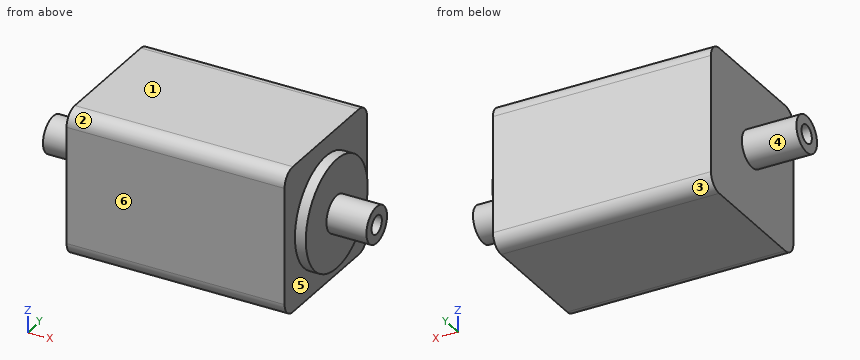
Autodesk Inventor part; units mm, degrees
ref_plane "Work Plane1" through (7, 10, -10) normal (1, 0, 0) x (0, 0, -1)
ref_plane "YZ Plane" through (0, 0, 0) normal (1, 0, 0) x (0, 1, 0)
ref_plane "XZ Plane" through (0, 0, 0) normal (0, 1, 0) x (-1, 0, 0)
sketch "Sketch1" plane through (0, 0, 0) normal (0, 1, 0) x (-1, 0, 0)
  line L0 (0, 0) -> (0, -20)
  line L1 (0, -20) -> (30, -20)
  line L2 (30, -20) -> (30, 0)
  line L3 (30, 0) -> (0, 0)
  dimension "d0" = 20
  dimension "d1" = 30
  dimension "d2" = 20
extrude "Extrusion1" add sketch "Sketch1" along normal blind 20
sketch "Sketch2" plane through (0, 0, 0) normal (1, 0, 0) x (0, 0, -1)
  line L0 (0, 0) -> (20, 0)
  line L1 (10, 0) -> (10, 10)
  circle A0 centre (10, 10) radius 7.5
  dimension "d5" = 10
  dimension "d6" = 15
extrude "Extrusion2" add sketch "Sketch2" along normal blind 1.5
sketch "Sketch3" plane through (1.5, 10, -10) normal (1, 0, 0) x (0, 0, -1)
  circle A0 centre (0, 0) radius 2.5
  point P0 (-10, -10)
  dimension "d9" = 5
extrude "Extrusion4" add sketch "Sketch3" along normal blind 5.5
sketch "Sketch4" plane through (-30, 0, -20) normal (-1, 0, 0) x (0, 0, 1)
  line L0 (20, 0) -> (0, 0)
  circle A0 centre (10, 10) radius 2.5
  circle A1 centre (10, 10) radius 2.5
  dimension "d16" = 5
extrude "Extrusion5" add sketch "Sketch4" along normal blind 7.5
sketch "Sketch5" plane through (-37.5, 10, -10) normal (-1, 0, 0) x (0, 0, 1)
  circle A0 centre (0, 0) radius 2.5
  point P0 (10, -10)
  dimension "d19" = 5
hole "Hole1" at (-37.5, 10, -10) direction (1, 0, 0) diameter 2.5 end through all
fillet "Fillet1" radius 2 4 edges at (-15, 20, -20) (-15, 20, 0) (-15, 0, -20) (-15, 0, 0)
ref_plane "Work Plane1" through (7, 10, -10) normal (1, 0, 0) x (0, 0, -1)
properties part number "NEMA8"
Read the model definition and answer for the solid it produces. Units are mm, in the model's axes. Face numbers are marked on the shaded views. A direction names the side the tool comes from. Give positions to 0.01 mm unless a question says otherwise; leave off trailing zeros. Loops run counter-clockwise (first coordinate to the right, second up) from the corner with the lowest first, then second, coordinate; pieces in that order, holes last.
Item 1: The part is cut by section D-D (y = 4). Write down the section's boundary in (x, z).
Item 2: The part is cut by section B-B (x = -26). Write down the section's boundary in (y, z), and give its area (3 significant figures).
Item 3: For the marked faces 4, 5 and 6, determine the directions among +Z, -Z, +X, -X, +Y, -Y from which every point of the face is accessible in a straight line to the end or side of a thin tool.
Item 4: The part is cut by section C-C (y = 10). Write down the section's boundary in (x, z), and give its area (3 significant figures).
Item 5: The mould has two halves that part along Y. Classify the marked faces 1, 2 and 3: released by +Y, released by -Y, zero draft, split by the parting line, or undercut.
Item 6: The part is cut by section A-A (z = -10). Write down the section's boundary in (x, y).
Item 7: Find the intervals of material crossed by line 1 along Y through (x, z) = (-9.5, -10); line 2 along Z through (x, y) = (-26, 10); line 3 along X through (y, z) = (4.5, -2), in increasing order.
Item 8: This flat-tipped pin is pushed along its axis until it touches: pin 1 Ø6 at (y, z) = (2.5, -8) entering from +X. Where does it stop, or does it pass through?
Taken from the geometry:
1. outline: (-30, -20) - (0, -20) - (0, -14.5) - (1.5, -14.5) - (1.5, -5.5) - (0, -5.5) - (0, 0) - (-30, 0) - close
2. outline: (0, -18) arc R2 ccw to (2, -20) - (18, -20) arc R2 ccw to (20, -18) - (20, -2) arc R2 ccw to (18, 0) - (2, 0) arc R2 ccw to (0, -2) - close; hole circle Ø2.5 at (10, -10)
2. area: 392 mm2
3. face 4: -X
3. face 5: +X
3. face 6: +Z, -Z, +X, -X, -Y
4. outline: (-37.5, -12.5) - (-30, -12.5) - (-30, -20) - (0, -20) - (0, -17.5) - (1.5, -17.5) - (1.5, -12.5) - (7, -12.5) - (7, -11.25) - (-37.5, -11.25) - close; (-37.5, -8.75) - (7, -8.75) - (7, -7.5) - (1.5, -7.5) - (1.5, -2.5) - (0, -2.5) - (0, 0) - (-30, 0) - (-30, -7.5) - (-37.5, -7.5) - close
4. area: 576 mm2
5. face 1: zero draft
5. face 2: released by -Y
5. face 3: released by +Y
6. outline: (-37.5, 7.5) - (-30, 7.5) - (-30, 0) - (0, 0) - (0, 2.5) - (1.5, 2.5) - (1.5, 7.5) - (7, 7.5) - (7, 8.75) - (-37.5, 8.75) - close; (-37.5, 11.25) - (7, 11.25) - (7, 12.5) - (1.5, 12.5) - (1.5, 17.5) - (0, 17.5) - (0, 20) - (-30, 20) - (-30, 12.5) - (-37.5, 12.5) - close
7. line 1: y = 0 to 8.75, 11.25 to 20
7. line 2: z = -20 to -11.25, -8.75 to 0
7. line 3: x = -30 to 0
8. pin 1: stops at x = 1.5
